Verification items for the finished model (mm, model axes). Round coordinates to 2 decimals unless told otherwise and drop trailing zeros. Loops run counter-clockwise (first coordinate to the right, second up) from the corner with the lowest first, then second, coordinate; pieces in that order, holes last. Notation, with made-up numbers: M -1.75,75 L 23.25,75 A13 ccw 23.25,88 Z; hole C 12.5,-37 d5. An arc over 180 degrees is marked long. One line per item, written item: value.
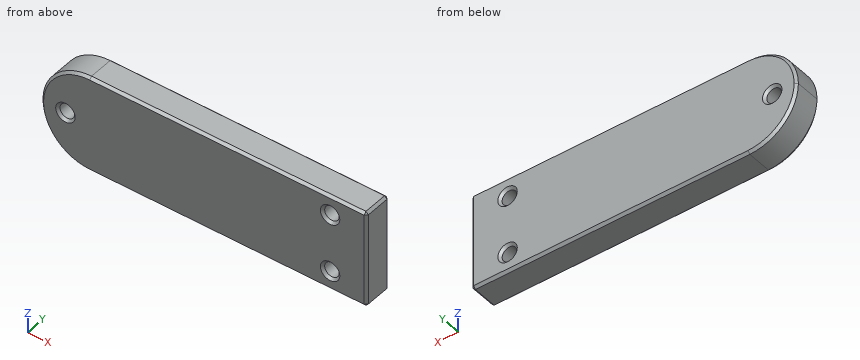
from build123d import *

# Parameters (mm, degrees)
CROQUIS1_W              = 67
CROQUIS1_H              = 20
CROQUIS1_R              = 1.5
SALIENTE_EXTRUIR1_DEPTH = 6
REDONDEO1_R             = 10
CHAFL_N2_SIZE           = 0.5


with BuildPart() as part:
    # Croquis1 → Saliente-Extruir1 (new body)
    with BuildSketch(Plane(origin=(0, 0, 0), x_dir=(1, 0, 0), z_dir=(0, 1, 0))):
        with Locations((28.5, 0)):
            Rectangle(CROQUIS1_W, CROQUIS1_H)
        with Locations(Location((0, 0, 0), (0, 0, 270))):
            Circle(CROQUIS1_R, mode=Mode.SUBTRACT)
        with Locations(Location((54.5, 6, 0), (0, 0, 270))):
            Circle(CROQUIS1_R, mode=Mode.SUBTRACT)
        with Locations(Location((54.5, -6, 0), (0, 0, 270))):
            Circle(CROQUIS1_R, mode=Mode.SUBTRACT)
    extrude(amount=SALIENTE_EXTRUIR1_DEPTH)

    # Redondeo1
    redondeo1_edges = [part.edges().sort_by_distance(p)[0] for p in [
        (-5, 3, -10),
        (-5, 3, 10),
    ]]
    fillet(redondeo1_edges, radius=REDONDEO1_R - 0.0001)  # a hair under: the kernel refuses the full size

    # Chaflán2
    chafl_n2_edges = [part.edges().sort_by_distance(p)[0] for p in [
        (0, 0, -1.5),
        (0, 6, -1.5),
        (54.5, 0, -7.5),
        (54.5, 6, -7.5),
        (54.5, 0, 4.5),
        (54.5, 6, 4.5),
        (33.49995, 0, 10),
        (-2.071097101, 0, 7.071097101),
        (-2.071097101, 0, -7.071097101),
        (33.49995, 6, 10),
        (-2.071097101, 6, 7.071097101),
        (-2.071097101, 6, -7.071097101),
        (62, 6, 0),
        (33.49995, 0, -10),
        (62, 0, 0),
        (33.49995, 6, -10),
        (62, 3, 10),
        (62, 3, -10),
    ]]
    chamfer(chafl_n2_edges, length=CHAFL_N2_SIZE)


solid = part.part
(1) Thickness scan on L1, parallel to Z at x = 55, y = 3.75; L2, parallel to Z at x = 53, y = 5.75; L3, parallel to X at y = 5.75, z = 1.5. Record the ranges inside material, lowest first. Write a range as from..to.
Completed:
L1: z = -10..-7.41, -4.59..4.59, 7.41..10
L2: z = -9.75..-6.9, -5.1..5.1, 6.9..9.75
L3: x = -4.63..-0.9, 0.9..61.75
(2) Sectioned sample at B-B on x = 54.5. Enter the section's corners in (y, z).
Completed:
outline: M 0,-9.5 L 0.5,-10 L 5.5,-10 L 6,-9.5 L 6,-8 L 5.5,-7.5 L 0.5,-7.5 L 0,-8 Z; M 0,-4 L 0.5,-4.5 L 5.5,-4.5 L 6,-4 L 6,4 L 5.5,4.5 L 0.5,4.5 L 0,4 Z; M 0,8 L 0.5,7.5 L 5.5,7.5 L 6,8 L 6,9.5 L 5.5,10 L 0.5,10 L 0,9.5 Z
(3) Sectioned sample at A-A on y = 3.25. Count the separate pieces of the cut face and the enclosed holes in it, and give its area (3 significant figures).
Completed:
separate pieces: 1
enclosed holes: 3
area: 1,280 mm^2
